Verification items for this drawing (mm, ordinates from the low corner). A direction names the side the tool comes from. Give positions to 0.01 mm unless a question says otherwise; leave off trailing zeros. Loops run counter-clockwise (first coordinate to the right, second up) from the corner with the lowest first, then second, coordinate; pieces in that order, holes last. Notation, with made-up numbers: (83.25, 31) -> (130.25, 31) arc R12 ccw to (130.25, 54) -> close; hole circle Ø8 at (49.5, -39.5). An arc over 180 degrees is marked (long way). Answer as CSV lines item,"result". Start each with the question number.
(1) Access from +Z, -Z, +X, -X, +Y, -Y to the whole of each face (thin tool, end or side, straight path). Record for the marked faces 1, 2 and 3.
(2) Section check A-A on x = 6.35. Enter the section's corners in (y, z).
(3) Material ranges on line 1 (Y direction, x = 4.5, z = 20); line 2 (X direction, y = 18.25, z = 12.5) (3 decimals); line 3 (Z direction, x = 2.75, y = 20.5), recorded low to high. Write a range as from..to.
(4) Gauge pin test, flat ends, axial feed: pin 1 Ø3 at (x, z) = (5.5, 18) entering from +Y; pin 2 Ø3 at (y, z) = (3, 3.5) entering from +X (1 decimal); pin 3 Ø1.1 at (y, z) = (19.5, 26) entering from -X (3 decimals). Record the tip position at first contact, or that the pin passes through.
(5) Section check B-B on z = 19.5. Enter the section's corners in (x, y) (1 decimal), plus the area to 3 significant figures.
(6) Section check D-D on x = 2.75. Enter the section's corners in (y, z), plus the area to 3 significant figures.
(7) Section check C-C on y = 23.25. Enter the section's corners in (x, z), plus the area to 3 significant figures.
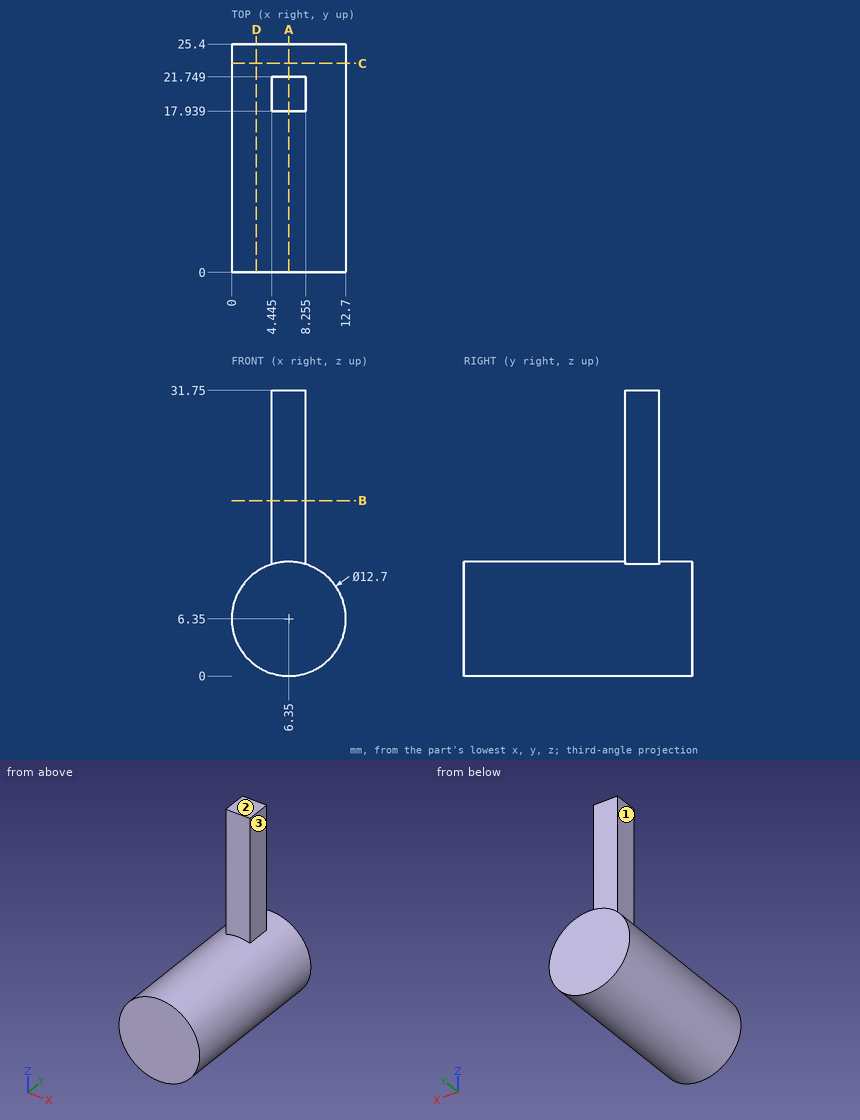
Working result:
1,face 1,"+Z, -X, +Y, -Y"
1,face 2,"+Z, +X, -X, +Y, -Y"
1,face 3,"+Z, +X, +Y, -Y"
2,outline,"(0, 0) -> (25.4, 0) -> (25.4, 12.7) -> (21.75, 12.7) -> (21.75, 31.75) -> (17.94, 31.75) -> (17.94, 12.7) -> (0, 12.7) -> close"
3,line 1,"y = 17.94..21.75"
3,line 2,"x = 4.445..8.255"
3,line 3,"z = 1.12..11.58"
4,pin 1,"stops at y = 21.75"
4,pin 2,"stops at x = 12.6"
4,pin 3,"stops at x = 4.445"
5,outline,"(4.4, 17.9) -> (8.3, 17.9) -> (8.3, 21.7) -> (4.4, 21.7) -> close"
5,area,"14.5 mm^2"
6,outline,"(0, 1.12) -> (25.4, 1.12) -> (25.4, 11.58) -> (0, 11.58) -> close"
6,area,"266 mm^2"
7,outline,"circle Ø12.7 at (6.35, 6.35)"
7,area,"127 mm^2"
